```python
from build123d import *

# Parameters (mm, degrees)
BOSS_EXTRUDE1_DEPTH = 5.969
CUT_EXTRUDE1_DEPTH  = 0.635
BOSS_EXTRUDE2_DEPTH = 5.969
FILLET4_R           = 1.524
FILLET5_R           = 2.54
FILLET3_R           = 0.254


with BuildPart() as part:
    # Sweep1: sweep along a path in Sketch1
    with BuildLine(Plane(origin=(0, 0, 0), x_dir=(1, 0, 0), z_dir=(0, 1, 0))) as sweep1_path:
        Line((-25.4, 28.575), (25.4, 28.575))
        ThreePointArc((25.4, 28.575), (27.64506403, 27.64506403), (28.575, 25.4))
        Line((28.575, 25.4), (28.575, -25.4))
        ThreePointArc((28.575, -25.4), (27.64506403, -27.64506403), (25.4, -28.575))
        Line((25.4, -28.575), (-25.4, -28.575))
        ThreePointArc((-25.4, -28.575), (-27.64506403, -27.64506403), (-28.575, -25.4))
        Line((-28.575, -25.4), (-28.575, 25.4))
        ThreePointArc((-28.575, 25.4), (-27.64506403, 27.64506403), (-25.4, 28.575))
    # Sketch2 → Sweep1 (sweep)
    with BuildSketch(Plane(origin=(0, 0, 0), x_dir=(0, 0, -1), z_dir=(1, 0, 0))):
        Polygon((27.051, 22.68081304), (29.337, 4.432166315), (29.337, 0), (26.035, 0), (26.035, 24.13), align=None)
    sweep(path=sweep1_path.line)

    # Sketch3 → Boss-Extrude1 (add)
    with BuildSketch(Plane.XZ):
        with BuildLine():
            Line((-25.4, -29.337), (0, -29.337))
            Line((0, -29.337), (25.4, -29.337))
            ThreePointArc((25.4, -29.337), (28.183879398, -28.183879398), (29.337, -25.4))
            Line((29.337, -25.4), (29.337, 25.4))
            ThreePointArc((29.337, 25.4), (28.183879398, 28.183879398), (25.4, 29.337))
            Line((25.4, 29.337), (-25.4, 29.337))
            ThreePointArc((-25.4, 29.337), (-28.183879398, 28.183879398), (-29.337, 25.4))
            Line((-29.337, 25.4), (-29.337, -25.4))
            ThreePointArc((-29.337, -25.4), (-28.183879398, -28.183879398), (-25.4, -29.337))
        make_face()
    extrude(amount=BOSS_EXTRUDE1_DEPTH)

    # Sketch4 → Cut-Extrude1 (cut)
    with BuildSketch(Plane.XZ.offset(5.969)):
        with BuildLine():
            Line((-25.4, -27.432), (25.4, -27.432))
            ThreePointArc((25.4, -27.432), (26.836840979, -26.836840979), (27.432, -25.4))
            Line((27.432, -25.4), (27.432, 25.4))
            ThreePointArc((27.432, 25.4), (26.836840979, 26.836840979), (25.4, 27.432))
            Line((25.4, 27.432), (-25.4, 27.432))
            ThreePointArc((-25.4, 27.432), (-26.836840979, 26.836840979), (-27.432, 25.4))
            Line((-27.432, 25.4), (-27.432, -25.4))
            ThreePointArc((-27.432, -25.4), (-26.836840979, -26.836840979), (-25.4, -27.432))
        make_face()
    extrude(amount=-CUT_EXTRUDE1_DEPTH, mode=Mode.SUBTRACT)

    # Sketch5 → Boss-Extrude2 (add)
    with BuildSketch(Plane.XZ.offset(5.969)):
        with BuildLine():
            Line((-33.147, 25.4), (-33.147, -25.4))
            ThreePointArc((-33.147, -25.4), (-30.877956234, -30.877956234), (-25.4, -33.147))
            Line((-25.4, -33.147), (25.4, -33.147))
            ThreePointArc((25.4, -33.147), (30.877956234, -30.877956234), (33.147, -25.4))
            Line((33.147, -25.4), (33.147, 25.4))
            ThreePointArc((33.147, 25.4), (30.877956234, 30.877956234), (25.4, 33.147))
            Line((25.4, 33.147), (-25.4, 33.147))
            ThreePointArc((-25.4, 33.147), (-30.877956234, 30.877956234), (-33.147, 25.4))
        make_face()
        with BuildLine():
            Line((-27.432, 25.4), (-27.432, -25.4))
            ThreePointArc((-27.432, -25.4), (-26.836840979, -26.836840979), (-25.4, -27.432))
            Line((-25.4, -27.432), (25.4, -27.432))
            ThreePointArc((25.4, -27.432), (26.836840979, -26.836840979), (27.432, -25.4))
            Line((27.432, -25.4), (27.432, 25.4))
            ThreePointArc((27.432, 25.4), (26.836840979, 26.836840979), (25.4, 27.432))
            Line((25.4, 27.432), (-25.4, 27.432))
            ThreePointArc((-25.4, 27.432), (-26.836840979, 26.836840979), (-27.432, 25.4))
        make_face(mode=Mode.SUBTRACT)
    extrude(amount=-BOSS_EXTRUDE2_DEPTH)

    # Fillet4
    fillet4_edges = [part.edges().sort_by_distance(p)[0] for p in [
        (0, 0, -29.337),
        (0, 0, -29.337),
        (-28.183879398, 0, -28.183879398),
        (-29.337, 0, 0),
        (-28.183879398, 0, 28.183879398),
        (0, 0, 29.337),
        (28.183879398, 0, 28.183879398),
        (29.337, 0, 0),
        (28.183879398, 0, -28.183879398),
    ]]
    fillet(fillet4_edges, radius=FILLET4_R)

    # Fillet5
    # the kernel refuses this fillet: 2.54 mm, written as the material it takes off along each edge
    with BuildSketch(Plane(origin=(-25.4, 0, -25.4), x_dir=(-1, 0, 0), z_dir=(0, 0, 1))) as fillet5_piece_1:
        with BuildLine():
            CenterArc((5.207, 2.532054733), FILLET5_R, 273.583321698, 86.416678302)
            Line((7.747, 2.532054733), (8.001, 2.532054733))
            Line((8.001, 2.532054733), (8.001, 0))
            Line((8.001, 0), (7.747, -0.254))
            ThreePointArc((7.747, -0.254), (5.461, -0.254), (5.381625, -0.256482896))
            Line((5.381625, -0.256482896), (5.36575, -0.002979475))
        make_face()
    revolve(axis=Axis((-25.4, 0, -25.4), (0, -1, 0)), revolution_arc=90, mode=Mode.SUBTRACT)
    with BuildSketch(Plane(origin=(-33.147, 0, 25.4), x_dir=(0.9999992172213047, 0.001251222113716365, 0), z_dir=(0, 0, -1)), Plane(origin=(25.4, 0, 33.147), x_dir=(0, 0.0012512221137164234, -0.9999992172213047), z_dir=(-1, 0, 0)), Plane(origin=(33.147, 0, -25.4), x_dir=(-0.9999992172213047, 0.0012512221137164405, 0), z_dir=(0, 0, 1)), Plane(origin=(-25.4, 0, -33.147), x_dir=(0, 0.001251222113716569, 0.9999992172213047), z_dir=(1, 0, 0))) as fillet5_piece_2:
        with BuildLine():
            CenterArc((2.536829849, 2.535230855), FILLET5_R, 180.071689765, 86.416678302)
            Line((-0.003168163, 2.532052751), (-0.257167964, 2.531734941))
            Line((-0.257167964, 2.531734941), (-0.253999801, -0.00031781))
            Line((-0.253999801, -0.00031781), (0.00031781, -0.253999801))
            ThreePointArc((0.00031781, -0.253999801), (2.286316021, -0.251139507), (2.365694066, -0.253523086))
            Line((2.365694066, -0.253523086), (2.381251864, 0))
        make_face()
    extrude(amount=50.8, mode=Mode.SUBTRACT)
    with BuildSketch(Plane(origin=(-25.4, 0, 25.4), x_dir=(0, 0, 1), z_dir=(1, 0, 0))) as fillet5_piece_3:
        with BuildLine():
            CenterArc((5.207, 2.532054733), FILLET5_R, 273.583321698, 86.416678302)
            Line((7.747, 2.532054733), (8.001, 2.532054733))
            Line((8.001, 2.532054733), (8.001, 0))
            Line((8.001, 0), (7.747, -0.254))
            ThreePointArc((7.747, -0.254), (5.461, -0.254), (5.381625, -0.256482896))
            Line((5.381625, -0.256482896), (5.36575, -0.002979475))
        make_face()
    revolve(axis=Axis((-25.4, 0, 25.4), (0, -1, 0)), revolution_arc=90, mode=Mode.SUBTRACT)
    with BuildSketch(Plane(origin=(25.4, 0, 25.4), x_dir=(1, 0, 0), z_dir=(0, 0, -1))) as fillet5_piece_4:
        with BuildLine():
            CenterArc((5.207, 2.532054733), FILLET5_R, 273.583321698, 86.416678302)
            Line((7.747, 2.532054733), (8.001, 2.532054733))
            Line((8.001, 2.532054733), (8.001, 0))
            Line((8.001, 0), (7.747, -0.254))
            ThreePointArc((7.747, -0.254), (5.461, -0.254), (5.381625, -0.256482896))
            Line((5.381625, -0.256482896), (5.36575, -0.002979475))
        make_face()
    revolve(axis=Axis((25.4, 0, 25.4), (0, -1, 0)), revolution_arc=90, mode=Mode.SUBTRACT)
    with BuildSketch(Plane(origin=(25.4, 0, -25.4), x_dir=(0, 0, -1), z_dir=(-1, 0, 0))) as fillet5_piece_5:
        with BuildLine():
            CenterArc((5.207, 2.532054733), FILLET5_R, 273.583321698, 86.416678302)
            Line((7.747, 2.532054733), (8.001, 2.532054733))
            Line((8.001, 2.532054733), (8.001, 0))
            Line((8.001, 0), (7.747, -0.254))
            ThreePointArc((7.747, -0.254), (5.461, -0.254), (5.381625, -0.256482896))
            Line((5.381625, -0.256482896), (5.36575, -0.002979475))
        make_face()
    revolve(axis=Axis((25.4, 0, -25.4), (0, -1, 0)), revolution_arc=90, mode=Mode.SUBTRACT)

    # Fillet3
    fillet3_edges = [part.edges().sort_by_distance(p)[0] for p in [
        (25.849012806, 24.13, 25.849012806),
        (0, 0, 26.035),
        (0, 24.13, 26.035),
        (-25.849012806, 0, 25.849012806),
        (-25.849012806, 24.13, 25.849012806),
        (0, 0, -26.035),
        (-26.035, 0, 0),
        (-26.035, 24.13, 0),
        (-25.849012806, 0, -25.849012806),
        (-25.849012806, 24.13, -25.849012806),
        (0, 0, -26.035),
        (0, 24.13, -26.035),
        (0, 24.13, -26.035),
        (25.849012806, 0, -25.849012806),
        (25.849012806, 24.13, -25.849012806),
        (26.035, 0, 0),
        (26.035, 24.13, 0),
        (25.849012806, 0, 25.849012806),
    ]]
    fillet(fillet3_edges, radius=FILLET3_R)


solid = part.part
```
Read the model definition and answer for the solid it produces. Units are mm, in the model's axes. A direction names the side the tool comes from. Give positions to 0.01 mm unless a question says otherwise; leave off trailing zeros. Write each loop counter-clockwise with the first axis right and the second up, starting at its lowest first coordinate (ties: lowest second). Pieces come first, ordered by that corner, then holes. Notation, with made-up numbers: (55.5, -26.75) - (93.5, -26.75) arc R19 cw to (93.5, -15.75) - close; hole circle Ø9 at (-31.75, -10.5). An arc over 180 degrees is marked (long way). Write item = value, one per line. Start each with the question number.
Item 1: The mould has two halves that part along Z. Classify faces 1 (the cylindrical face through (-26.853, -5.656, -26.821)), 2 (the cylindrical face through (30.817, -4.275, -30.938)), 3 (the flat face through (0, 12, -26.035)), 4 (the flat face through (-28.21, 13.43, -0.36)): +Z half, -Z half, draft (parallel to the pull), parting line (faces both ways), or undercut.
Item 2: A tool of negligible diameter and unlimited length cuts with its end or side. For faces 5 (the cylindrical face through (-32.477, -0.813, 0.356)), 6 (the cylindrical face through (26.853, -5.656, 26.821)), 7 (the cylindrical face through (-28.153, 2.998, 28.214)), from which of +Z, -Z, +X, -X, +Y, -Y can it reach the whole face along a straight path? Write none if from no direction.
Item 3: Find section C-C (x = 20). Give the vertices of the cut face in (y, z) (3 decimals).
Item 4: Find section B-B (y = 6). Give the vertices of the cut face in (x, z) (3 decimals).
Item 5: Find the intervals of material crossed by probe 1 along Z at (x, y) = (-3.5, 4) (3 decimals); probe 2 along X at (y, z) = (8.75, 5.5) (3 decimals); probe 3 along Z at (x, y) = (8, 6) (3 decimals), in increasing order. Write a range as [from, to].
Item 6: Each of these flat-tipped pins is pushed along its axis until it touches: P1, Ø11.5, axis at y = 7, z = 1, coming from the -X side; P2, Ø15.5, axis at x = 3, z = 5.5, coming from the +Y side; P3, Ø11.5, axis at x = 12, y = 11, coming from the -Z side. Where does it stop, or does it pass through?
Item 7: Find section A-A (z = 12). Give the vertices of the cut face in (x, y) (3 decimals), then the cut area to 3 significant figures.
Item 8: Find section D-D (y = 16.5). Give the vertices of the cut face in (x, z) (3 decimals).
Response:
q1.face_1 = undercut
q1.face_2 = -Z half
q1.face_3 = undercut
q1.face_4 = draft
q2.face_5 = +Z, -Z, -X, +Y
q2.face_6 = -Y
q2.face_7 = +Z, -X, +Y
q3.outline = (-5.969, -33.147) - (-2.532, -33.147) arc R2.54 ccw to (0.003, -30.766) arc R1.524 cw to (1.524, -29.337) - (4.432, -29.337) - (22.681, -27.051) - (23.471, -26.497) arc R0.254 ccw to (23.325, -26.035) - (0.254, -26.035) arc R0.254 cw to (0, -25.781) - (0, 25.781) arc R0.254 cw to (0.254, 26.035) - (23.325, 26.035) arc R0.254 ccw to (23.471, 26.497) - (22.681, 27.051) - (4.432, 29.337) - (1.524, 29.337) arc R1.524 cw to (0.003, 30.766) arc R2.54 ccw to (-2.532, 33.147) - (-5.969, 33.147) - (-5.969, 27.432) - (-5.334, 27.432) - (-5.334, -27.432) - (-5.969, -27.432) - close
q4.outline = (-29.141, -25.4) arc R3.741 ccw to (-25.4, -29.141) - (25.4, -29.141) arc R3.741 ccw to (29.141, -25.4) - (29.141, 25.4) arc R3.741 ccw to (25.4, 29.141) - (-25.4, 29.141) arc R3.741 ccw to (-29.141, 25.4) - close; hole (-26.035, -25.4) arc R0.635 ccw to (-25.4, -26.035) - (25.4, -26.035) arc R0.635 ccw to (26.035, -25.4) - (26.035, 25.4) arc R0.635 ccw to (25.4, 26.035) - (-25.4, 26.035) arc R0.635 ccw to (-26.035, 25.4) - close
q5.probe_1 = [-29.337, -26.035], [26.035, 29.337]
q5.probe_2 = [-28.796, -26.035], [26.035, 28.796]
q5.probe_3 = [-29.141, -26.035], [26.035, 29.141]
q6.P1 = -29.36
q6.P2 = 0
q6.P3 = -29.23
q7.outline = (-33.147, -5.969) - (-27.432, -5.969) - (-27.432, -5.334) - (27.432, -5.334) - (27.432, -5.969) - (33.147, -5.969) - (33.147, -2.532) arc R2.54 ccw to (30.766, 0.003) arc R1.524 cw to (29.337, 1.524) - (29.337, 4.432) - (27.051, 22.681) - (26.497, 23.471) arc R0.254 ccw to (26.035, 23.325) - (26.035, 0.254) arc R0.254 cw to (25.781, 0) - (-25.781, 0) arc R0.254 cw to (-26.035, 0.254) - (-26.035, 23.325) arc R0.254 ccw to (-26.497, 23.471) - (-27.051, 22.681) - (-29.337, 4.432) - (-29.337, 1.524) arc R1.524 cw to (-30.766, 0.003) arc R2.54 ccw to (-33.147, -2.532) - close
q7.area = 468 mm²
q8.outline = (-27.825, -25.4) arc R2.425 ccw to (-25.4, -27.825) - (25.4, -27.825) arc R2.425 ccw to (27.825, -25.4) - (27.825, 25.4) arc R2.425 ccw to (25.4, 27.825) - (-25.4, 27.825) arc R2.425 ccw to (-27.825, 25.4) - close; hole (-26.035, -25.4) arc R0.635 ccw to (-25.4, -26.035) - (25.4, -26.035) arc R0.635 ccw to (26.035, -25.4) - (26.035, 25.4) arc R0.635 ccw to (25.4, 26.035) - (-25.4, 26.035) arc R0.635 ccw to (-26.035, 25.4) - close
